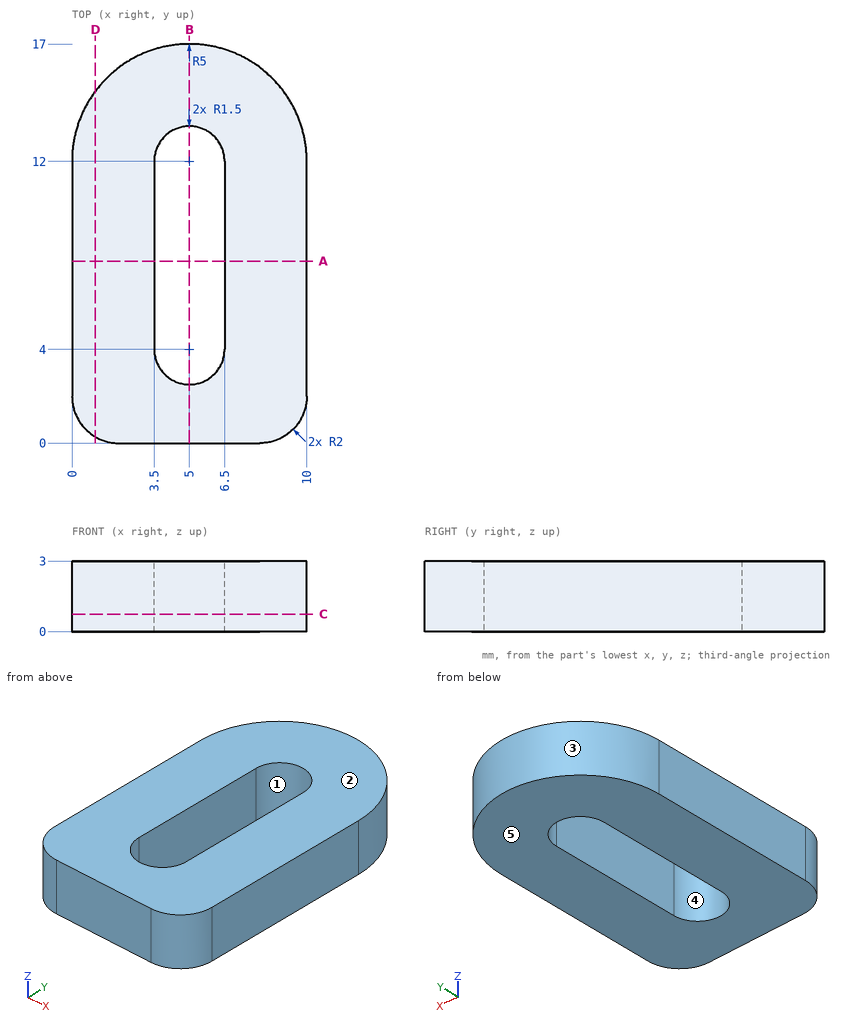
The figure shows three views and two pictorial views of one solid part (mm, origin at its lowest corner). Answer the questions. A direction names the side the tool comes from. Round coordinates to 2 decimals unless told otherwise and drop trailing zeros. Write each loop counter-clockwise with the first axis right and the second up, starting at its lowest first coordinate (ties: lowest second). Pieces come first, ordered by that corner, then holes. Notation, with made-up numbers: M 72.5,-3 L 109.5,-3 A13 ccw 109.5,19 Z; hole C 4,-34 d5. An arc over 180 degrees is marked long. Use a Markdown table: item, result.
1) Consider line 1 (X direction, y = 10, z = 2.3); line 2 (Y direction, x = 5, z = 1.85); line 3 (X direction, y = 12.5, z = 1.3). Determine where each line is inside the solid, lowest interval first. Write a range as [from, to].
Taken from the geometry:
| item | result |
|---|---|
| line 1 | x = [0, 3.5], [6.5, 10] |
| line 2 | y = [0, 2.5], [13.5, 17] |
| line 3 | x = [0.03, 3.59], [6.41, 9.97] |
2) A flat-ended cylindrical pin translates along its axis: pin 1 (0.9 mm diameter, centred on y = 10, z = 1, fed in from -X). Find the tip coordinate at first contact, or state that the pin passes through.
Taken from the geometry:
| item | result |
|---|---|
| pin 1 | stops at x = 0 |
3) The part is cut by section D-D on x = 1. Give the vertices of the cut face in (y, z).
Taken from the geometry:
| item | result |
|---|---|
| outline | M 0.27,0 L 15,0 L 15,3 L 0.27,3 Z |
4) Which of the six approach directions +Z, -Z, +X, -X, +Y, -Y give full straight-line access (tool end or side, diameter ignored) to the marked faces 4 and 5?
Taken from the geometry:
| item | result |
|---|---|
| face 4 | +Z, -Z |
| face 5 | -Z, +X, -X, +Y, -Y |
5) Determine the mould class of the marked faces 1, 2 and 3 for opening direction Y: pulls with the +Y half, pulls with the -Y half, needs draft (parallel to the pull), parting line crosses it, or undercut.
Taken from the geometry:
| item | result |
|---|---|
| face 1 | undercut |
| face 2 | needs draft |
| face 3 | pulls with the +Y half |
6) The part is cut by section A-A on y = 7.75. Give the vertices of the cut face in (x, z), plus the area to 3 significant figures.
Taken from the geometry:
| item | result |
|---|---|
| outline | M 0,0 L 3.5,0 L 3.5,3 L 0,3 Z; M 6.5,0 L 10,0 L 10,3 L 6.5,3 Z |
| area | 21.0 mm2 |
7) The part is cut by section C-C on z = 0.75. Give the vertices of the cut face in (x, y), plus the area to 3 significant figures.
Taken from the geometry:
| item | result |
|---|---|
| outline | M 0,2 A2 ccw 2,0 L 8,0 A2 ccw 10,2 L 10,12 A5 ccw 0,12 Z; hole M 3.5,4 A1.5 ccw 6.5,4 L 6.5,12 A1.5 ccw 3.5,12 Z |
| area | 126 mm2 |
8) The part is cut by section B-B on x = 5. Give the vertices of the cut face in (y, z), plus the area to 3 significant figures.
Taken from the geometry:
| item | result |
|---|---|
| outline | M 0,0 L 2.5,0 L 2.5,3 L 0,3 Z; M 13.5,0 L 17,0 L 17,3 L 13.5,3 Z |
| area | 18.0 mm2 |
